Here's how the part is built. I have some questions about the finished solid (model axes, mm). Coordinates: 2 decimals unless noted, no trailing zeros. Write each loop counter-clockwise with the first axis right and the second up, starting at its lowest first coordinate (ties: lowest second). Pieces come first, ordered by that corner, then holes.
Item 1: If we section it at D-D (x = 8.5): Please give me the cut outline in (y, z), then the cut area to 3 significant figures.
Item 2: I'm going to push flat-ended pins straight in: pin 1 Ø11 at (x, z) = (0, 0) entering from -Y; pin 2 Ø10 at (x, z) = (-6.5, -45.5) entering from -Y. Where does each tip first touch, or does it pass through?
Item 3: If we section it at A-A (z = 31.75): Please give me the cut outline in (x, y) (3 decimals).
Item 4: If we section it at B-B (x = 0): Please give me the cut outline in (y, z) (3 decimals).
Item 5: If I drill on line 1 (Z direction, x = 0, y = 3.75) (3 decimals); line 2 (Z direction, x = 4, y = 1.5); line 3 (X direction, y = 4.25, z = 1), over which ranges is the centre line in solid material (lowest first)?
Item 6: If we section it at C-C (y = 2.75): Please give me the cut outline in (x, z) (3 decimals), then the cut area to 3 significant figures.
Item 7: We'd pull the mould along X, two halves only. Please class faces 1 (the face through (0.909, 3.131, -6.926)), 2 (the face through (1.51, 3.13, 38.57)), 3 (the face through (-0.419, 3.131, -57.145)), 4 (the face through (9, 0, 1)): +X half, -X half, draft (parallel to the pull), parting line (faces both ways), or undercut.
Autodesk Inventor part; units mm, degrees
ref_plane "YZ Plane" through (0, 0, 0) normal (1, 0, 0) x (0, 1, 0)
ref_plane "XZ Plane" through (0, 0, 0) normal (0, 1, 0) x (-1, 0, 0)
ref_plane "XY Plane" through (0, 0, 0) normal (0, 0, 1) x (1, 0, 0)
sketch "Sketch1" plane through (0, 0, 0) normal (0, 1, 0) x (-1, 0, 0)
  line L0 (0, -38.1) -> (0, 38.1) construction
  line L1 (19.05, -38.1) -> (19.05, 38.1)
  line L2 (-19.05, 38.1) -> (-19.05, -38.1)
  arc A0 (-19.05, -38.1) -> (19.05, -38.1) centre (0, -38.1) ccw
  arc A1 (19.05, 38.1) -> (-19.05, 38.1) centre (0, 38.1) ccw
  circle A2 centre (0, 0) radius 6.985
  circle A3 centre (0, -31.75) radius 6.985
  circle A4 centre (0, 31.75) radius 6.985
  line L3 (34.1256, 57.15) -> (-20.0171, 57.15)
  line L4 (24.6444, -57.15) -> (-26.3115, -57.15)
  dimension "d0" = 38.1
  dimension "d1" = 38.1
  dimension "d2" = 13.97
  dimension "d3" = 31.75
  dimension "d4" = 31.75
  dimension "d7" = 114.3
extrude "Extrusion1" add sketch "Sketch1" along normal blind 6.35
properties part number "Top Panel"
Answer list:
1. outline: (0, -55.15) - (6.35, -55.15) - (6.35, 55.15) - (0, 55.15) - close
1. area: 700 mm2
2. pin 1: passes through
2. pin 2: stops at y = 0
3. outline: (-19.05, 0) - (-6.985, 0) - (-6.985, 6.35) - (-19.05, 6.35) - close; (6.985, 0) - (19.05, 0) - (19.05, 6.35) - (6.985, 6.35) - close
4. outline: (0, -57.15) - (6.35, -57.15) - (6.35, -38.735) - (0, -38.735) - close; (0, -24.765) - (6.35, -24.765) - (6.35, -6.985) - (0, -6.985) - close; (0, 6.985) - (6.35, 6.985) - (6.35, 24.765) - (0, 24.765) - close; (0, 38.735) - (6.35, 38.735) - (6.35, 57.15) - (0, 57.15) - close
5. line 1: z = -57.15 to -38.735, -24.765 to -6.985, 6.985 to 24.765, 38.735 to 57.15
5. line 2: z = -56.73 to -37.48, -26.02 to -5.73, 5.73 to 26.02, 37.48 to 56.73
5. line 3: x = -19.05 to -6.91, 6.91 to 19.05
6. outline: (-19.05, -38.1) arc R19.05 ccw to (19.05, -38.1) - (19.05, 38.1) arc R19.05 ccw to (-19.05, 38.1) - close; hole circle Ø13.97 at (0, -31.75); hole circle Ø13.97 at (0, 0); hole circle Ø13.97 at (0, 31.75)
6. area: 3,580 mm2
7. face 1: undercut
7. face 2: undercut
7. face 3: parting line
7. face 4: draft
